from build123d import *

# Parameters (mm, degrees)
F0_R     = 7
F0_R_2   = 5
F1_DEPTH = 76.2
F0_R_3   = 1.5
F2_DEPTH = 3
F3_R     = 1.99999


# Not quite as in the source:
# - a fillet or chamfer is up to 0.001 mm smaller than in the source, because OpenCascade refuses the exact size


with BuildPart() as f1:
    # F0 (on Top) → F1 (new body)
    with BuildSketch(Plane.XY):
        Circle(F0_R)
        Circle(F0_R_2, mode=Mode.SUBTRACT)
    extrude(amount=F1_DEPTH)

    # F0 (on Top) → F2 (join)
    with BuildSketch(Plane.XY):
        Circle(F0_R)
        Circle(F0_R_2, mode=Mode.SUBTRACT)
        Circle(F0_R_2)
        Circle(F0_R_3, mode=Mode.SUBTRACT)
    extrude(amount=-F2_DEPTH)

    # F3 (radius 2 in the source; OpenCascade refuses exactly that, so slightly less here)
    f3_edges = [f1.edges().sort_by_distance(p)[0] for p in [
        (-7, 0, 76.2),
    ]]
    fillet(f3_edges, radius=F3_R)


solid = f1.part
Design review of the part built by this model. Coordinates are the model's own, in mm. A direction names the side the tool comes from. Coordinates: 2 decimals unless noted, no trailing zeros. Loops run counter-clockwise (first coordinate to the right, second up) from the corner with the lowest first, then second, coordinate; pieces in that order, holes last. Notation, with made-up numbers: (-2, -17) - (57, -17) arc R16 cw to (57, -10) - close; hole circle Ø9 at (-25, 42.5). An arc over 180 degrees is marked (long way). Use CSV: the item, a comma, the result in double quotes. Start each with the question number.
1. Mouldability with a two-part tool opening along X and no side actions: class faces 1 (the cylindrical face through (-1.08, -4.88, 37.57)), 2 (the flat face through (0, 2, -3)), 3 (the cylindrical face through (6.466, -2.681, 36.14)) as released by +X, released by -X, zero draft, split by the parting line, or undercut.
2. To check wall thickness, follow probe 1 along Y at (x, z) = (0, 14); probe 2 along Y at (x, z) = (0, -1.8); probe 3 along X at (y, z) = (-4.25, 15). State the ranges of each line that lie inside material, in increasing order.
3. Clearance check with flat-ended pins moving along their axes: pin 1 (1 mm diameter, centred on x = 1.5, z = 46, fed in from -Y); pin 2 (1.5 mm diameter, centred on y = 2.5, z = 26, fed in from +X); pin 3 (8 mm diameter, centred on x = 0.5, y = -0.5, fed in from +Z). State where each tip first meets the part, or that it passes through.
4. For faces 4 (the flat face through (-1.2, 1.2, 0)), 5 (the cylindrical face through (-1.5, 0.07, -1.48)), list the 3-axis set-ups (+Z, -Z, +X, -X, +Y, -Y) from which the entire face can be reached by the end or side of a thin tool; tool diameter is ignored.
5. Add section C-C on z = 60.5. Give the boundary of the cut face in (x, y), plus the area to 3 significant figures.
Resolved:
1,face 1,"undercut"
1,face 2,"zero draft"
1,face 3,"split by the parting line"
2,probe 1,"-7 to -5, 5 to 7"
2,probe 2,"-7 to -1.5, 1.5 to 7"
2,probe 3,"-5.56 to -2.63, 2.63 to 5.56"
3,pin 1,"y = -6.93"
3,pin 2,"x = 6.78"
3,pin 3,"z = 0"
4,face 4,"+Z"
4,face 5,"+Z, -Z"
5,outline,"circle Ø14 at (0, 0); hole circle Ø10 at (0, 0)"
5,area,"75.4 mm2"
